Here's how the part is built. I have some questions about the finished solid (model axes, mm). A direction names the side the tool comes from. Round coordinates to 2 decimals unless told otherwise and drop trailing zeros. Write each loop counter-clockwise with the first axis right and the second up, starting at its lowest first coordinate (ties: lowest second). Pieces come first, ordered by that corner, then holes. Notation, with made-up numbers: M -33,35.5 L 16,35.5 A12 cw 16,45.5 Z; hole C -29.5,69 d7. An arc over 180 degrees is marked long. Use a Markdown table: item, result. Add a question column.
```python
from build123d import *

# Parameters (mm, degrees)
F1_DEPTH = 25
F2_R     = 5
F3_DEPTH = 12.5
F4_R     = 4.5
F5_DEPTH = 3.201
F6_R     = 5


with BuildPart() as f1:
    # F0 (on Front) → F1 (new body)
    with BuildSketch(Plane.XZ):
        with BuildLine():
            Line((0, 3.2), (0, 0))
            Line((0, 0), (93.8, 0))
            ThreePointArc((93.8, 0), (98.184062, 1.815938), (100, 6.2))
            Line((100, 6.2), (100, 50))
            Line((100, 50), (96.8, 50))
            Line((96.8, 50), (96.8, 6.2))
            ThreePointArc((96.8, 6.2), (95.92132, 4.07868), (93.8, 3.2))
            Line((93.8, 3.2), (0, 3.2))
        make_face()
    extrude(amount=F1_DEPTH)

    # F2 (on face) → F3 (cut, symmetric)
    with BuildSketch(Plane(origin=(96.8, 0, 0), x_dir=(0, -1, 0), z_dir=(-1, 0, 0))):
        with Locations((12.5, 40)):
            Circle(F2_R)
    extrude(amount=F3_DEPTH, both=True, mode=Mode.SUBTRACT)

    # F4 (on face) → F5 (cut, through all)
    with BuildSketch(Plane.XY.offset(3.2)):
        with Locations((15, -12.5)):
            Circle(F4_R)
    extrude(amount=-F5_DEPTH, mode=Mode.SUBTRACT)

    # F6
    f6_edges = [f1.edges().sort_by_distance(p)[0] for p in [
        (0, -25, 1.6),
        (0, 0, 1.6),
        (98.4, 0, 50),
        (98.4, -25, 50),
    ]]
    fillet(f6_edges, radius=F6_R)


solid = f1.part
```
Item 1: On a 3-axis mill with a long thin cutter (end or side, diameter ignored), from which of +Z, -Z, +X, -X, +Y, -Y can I reach the whole of each face in a straight line? I mean faces 1 (the face through (48, -12, 3.2)), 2 (the face through (66, 0, 3)). Say none if no direction works.
Item 2: Imagine slicing it at A-A on z = 40. List the corners of the cut face in (x, y) for me.
Item 3: If we mould it in two halves opening along Y, with no side actions, what happens to faces 3 (the face through (98, -12, 50)), 4 (the face through (1, -2, 2)), 5 (the face through (10.504, -12.302, 1.622))? For each: +Y half, -Y half, draft (parallel to the pull), parting line (faces both ways), or undercut.
Item 4: I need wall thicknesses on probe 1 along X at (y, z) = (-1.25, 48); probe 2 along Z at (x, y) = (79, -21); probe 3 along Z at (x, y) = (97.9, -12.5). Which ranges of each line are inside material? Lowest first, please. Write a range as from..to.
Item 5: Imagine slicing it at B-B on y = -12.5. List the corners of the cut face in (x, z) for me, plus the area to 3 significant figures.
Item 6: Imagine slicing it at D-D on y = -2. List the corners of the cut face in (x, z) for me.
Item 7: For pin 1 Ø4 at (y, z) = (-4.5, 29.5) entering from -X; pin 2 Ø5 at (x, y) = (70, -3) entering from +Z; pin 3 Ø12 at (y, z) = (-12.5, 11) entering from -X, each with a flat end and sliding along its axis, tell me the tip position at first contact or that it passes through.
Item 8: Imagine slicing it at C-C on x = 15. List the corners of the cut face in (y, z) for me, plus the area to 3 significant figures.
The answers:
| question | item | result |
|---|---|---|
| 1 | face 1 | +Z, -X, +Y, -Y |
| 1 | face 2 | +Z, -Z, +X, -X, +Y |
| 2 | outline | M 96.8,-25 L 100,-25 L 100,-17.5 L 96.8,-17.5 Z; M 96.8,-7.5 L 100,-7.5 L 100,0 L 96.8,0 Z |
| 3 | face 3 | draft |
| 3 | face 4 | +Y half |
| 3 | face 5 | undercut |
| 4 | probe 1 | 96.8..100 |
| 4 | probe 2 | 0..3.2 |
| 4 | probe 3 | 1.55..35, 45..50 |
| 5 | outline | M 0,0 L 10.5,0 L 10.5,3.2 L 0,3.2 Z; M 19.5,0 L 93.8,0 A6.2 ccw 100,6.2 L 100,35 L 96.8,35 L 96.8,6.2 A3 cw 93.8,3.2 L 19.5,3.2 Z; M 96.8,45 L 100,45 L 100,50 L 96.8,50 Z |
| 5 | area | 403 mm² |
| 6 | outline | M 1,0 L 93.8,0 A6.2 ccw 100,6.2 L 100,49 L 96.8,49 L 96.8,6.2 A3 cw 93.8,3.2 L 1,3.2 Z |
| 7 | pin 1 | x = 96.8 |
| 7 | pin 2 | z = 3.2 |
| 7 | pin 3 | x = 96.55 |
| 8 | outline | M -25,0 L -17,0 L -17,3.2 L -25,3.2 Z; M -8,0 L 0,0 L 0,3.2 L -8,3.2 Z |
| 8 | area | 51.2 mm² |
